from build123d import *

# Parameters (mm, degrees)
F1_DEPTH = 1000


with BuildPart() as f1:
    # F0 (on Top) → F1 (new body)
    with BuildSketch(Plane.XY):
        Polygon((-5, 30.5), (-5, 32), (-10, 32), (-10, -32), (-5, -32), (-5, -30.5), (-8.5, -30.5), (-8.5, -26), (8.5, -26), (8.5, -30.5), (5, -30.5), (5, -32), (10, -32), (10, 32), (5, 32), (5, 30.5), (8.5, 30.5), (8.5, 26), (-8.5, 26), (-8.5, 30.5), align=None)
        Polygon((-8.5, 9.5), (-8.5, 24.5), (8.5, 24.5), (8.5, 9.5), (5.5, 9.5), (5.5, 7.5), (8.5, 7.5), (8.5, -7.5), (5.5, -7.5), (5.5, -9.5), (8.5, -9.5), (8.5, -24.5), (-8.5, -24.5), (-8.5, -9.5), (-5.5, -9.5), (-5.5, -7.5), (-8.5, -7.5), (-8.5, 7.5), (-5.5, 7.5), (-5.5, 9.5), align=None, mode=Mode.SUBTRACT)
    extrude(amount=F1_DEPTH)


solid = f1.part
Can you work these out from the model? Positions are in its coordinate system, mm. A direction names the side the tool comes from. Give positions to 0.01 mm unless a question says otherwise; leave off trailing zeros. Order: outer loops, then holes, each group sorted by start corner. A loop starts at its lowest first (then second) coordinate and runs counter-clockwise, first axis right, second up. Notation, with made-up numbers: M -8,85.25 L 46,85.25 A21 cw 46,102.25 Z; hole C 70,72.5 d9. An arc over 180 degrees is marked long. Use one line per item in the form item = value. Start each with the question number.
Item 1: We'd pull the mould along Y, two halves only. Please class faces 3 (the flat face through (0, -24.5, 493)), 4 (the flat face through (10, 0, 493)): +Y half, -Y half, draft (parallel to the pull), parting line (faces both ways), or undercut.
Item 2: If we section it at A-A (x = -1): Write out the boundary of the cut face in (y, z).
Item 3: If I drill on line 1 along Y through (x, z) = (-8.25, 711.5); line 2 along Y through (x, z) = (-5.25, 696); line 3 along X through (y, z) = (-0.5, 770), over which ranges is the centre line in solid material (lowest first)?
Item 4: For faces 1 (the flat face through (7, -9, 1000)), 2 (the flat face through (0, -26, 493)), which set-ups out of +Z, -Z, +X, -X, +Y, -Y let a thin tool reach every point of the face, with its end or its side?
Item 5: Will these pins go through, and if not, where does the flat tip stop? pin 1 Ø3 at (x, z) = (4, 835.5) entering from -Y; pin 2 Ø2 at (x, y) = (6, -19) entering from -Z; pin 3 Ø1.5 at (x, z) = (-1.5, 333.5) entering from -Y.
Outcome:
q1.face_3 = undercut
q1.face_4 = draft
q2.outline = M -26,0 L -24.5,0 L -24.5,1000 L -26,1000 Z; M 24.5,0 L 26,0 L 26,1000 L 24.5,1000 Z
q3.line_1 = -32 to -30.5, -26 to -24.5, -9.5 to -7.5, 7.5 to 9.5, 24.5 to 26, 30.5 to 32
q3.line_2 = -32 to -30.5, -26 to -24.5, 24.5 to 26, 30.5 to 32
q3.line_3 = -10 to -8.5, 8.5 to 10
q4.face_1 = +Z, +X, -X, +Y, -Y
q4.face_2 = +Z, -Z
q5.pin_1 = -32
q5.pin_2 = through
q5.pin_3 = -26
